```python
from build123d import *

# Parameters (mm, degrees)
MAIN_FEATURES_SKETCH_W   = 70.04
MAIN_FEATURES_SKETCH_H   = 57.05
MAIN_BODY_DEPTH          = 27.3
WIRES_START              = 2.1
MAIN_FEATURES_SKETCH_3_W = 4
MAIN_FEATURES_SKETCH_3_H = 10
WIRES_2_DEPTH            = 4
LENS_CUTOUT_START        = 27.3
MAIN_FEATURES_SKETCH_4_W = 50
MAIN_FEATURES_SKETCH_4_H = 37
LENS_CUTOUT_DEPTH        = 3.1
MAIN_FEATURES_SKETCH_5_R = 2.25
SCREW_HEADS_DEPTH        = 0.3
FILLET1_R                = 1
FILLET2_R                = 2


with BuildPart() as part:
    # main_features_sketch → main_body (new body)
    with BuildSketch(Plane.XY):
        Rectangle(MAIN_FEATURES_SKETCH_W, MAIN_FEATURES_SKETCH_H)
    extrude(amount=MAIN_BODY_DEPTH)

    # main_features_sketch<3> → wires 2 (add)
    with BuildSketch(Plane.XY.offset(WIRES_START)):
        with Locations((-18, -33.525)):
            Rectangle(MAIN_FEATURES_SKETCH_3_W, MAIN_FEATURES_SKETCH_3_H)
        with Locations((18, -33.525)):
            Rectangle(MAIN_FEATURES_SKETCH_3_W, MAIN_FEATURES_SKETCH_3_H)
    extrude(amount=WIRES_2_DEPTH)

    # main_features_sketch<4> → lens_cutout (cut)
    with BuildSketch(Plane.XY.offset(LENS_CUTOUT_START)):
        Rectangle(MAIN_FEATURES_SKETCH_4_W, MAIN_FEATURES_SKETCH_4_H)
    extrude(amount=-LENS_CUTOUT_DEPTH, mode=Mode.SUBTRACT)

    # main_features_sketch<5> → screw_heads (add)
    with BuildSketch(Plane.XY):
        with Locations((-32, -25.5)):
            Circle(MAIN_FEATURES_SKETCH_5_R)
        with Locations((32, -25.5)):
            Circle(MAIN_FEATURES_SKETCH_5_R)
        with Locations((32, 25.5)):
            Circle(MAIN_FEATURES_SKETCH_5_R)
        with Locations((-32, 25.5)):
            Circle(MAIN_FEATURES_SKETCH_5_R)
    extrude(amount=-SCREW_HEADS_DEPTH)

    # Fillet1
    fillet1_edges = [part.edges().sort_by_distance(p)[0] for p in [
        (35.02, 28.525, 13.65),
        (35.02, -28.525, 13.65),
        (-35.02, -28.525, 13.65),
        (-35.02, 28.525, 13.65),
    ]]
    fillet(fillet1_edges, radius=FILLET1_R)

    # Fillet2
    fillet2_edges = [part.edges().sort_by_distance(p)[0] for p in [
        (20, -33.525, 2.1),
        (20, -33.525, 6.1),
        (16, -33.525, 2.1),
        (16, -33.525, 6.1),
        (-16, -33.525, 2.1),
        (-16, -33.525, 6.1),
        (-20, -33.525, 2.1),
        (-20, -33.525, 6.1),
    ]]
    fillet(fillet2_edges, radius=FILLET2_R - 0.0001)  # a hair under: the kernel refuses the full size


solid = part.part
```
For this review, take the finished solid that the model builds, in its own axes (mm). A direction names the side the tool comes from. Coordinates: 2 decimals unless noted, no trailing zeros. Order: outer loops, then holes, each group sorted by start corner. A loop starts at its lowest first (then second) coordinate and runs counter-clockwise, first axis right, second up. Notation, with made-up numbers: (25.25, -4) - (62.25, -4) arc R21 ccw to (62.25, 24) - close; hole circle Ø4 at (61, -13). An arc over 180 degrees is marked (long way). Answer as a JSON object with one key per item and string values. Group by question number.
1. We need section B-B on x = 1. State the section outline as (y, z) points (3 decimals).
2. We need section C-C on z = 10. State the section outline as (x, y) points (3 decimals).
3. We need section D-D on x = -32. State the section outline as (y, z) points (3 decimals).
4. For probe 1 along Y at (x, z) = (-15, 24.25) (3 decimals); probe 2 along Z at (x, y) = (-22, 7.5); probe 3 along Y at (x, z) = (17.5, 16) (3 decimals), list the stretches that pass through material, from the lowest coordinate up.
5. For faces 1 (the flat face through (0, 0, 0)), 2 (the flat face through (0, 0, 24.2)), 3 (the cylindrical face through (19.43, -33.46, 2.7)), 4 (the cylindrical face through (-16.57, -33.46, 2.7)), list the 3-axis set-ups (+Z, -Z, +X, -X, +Y, -Y) from which the entire face can be reached by the end or side of a thin tool; tool diameter is ignored.
6. Clearance check with flat-ended pins moving along their axes: P1, Ø10, axis at x = 12, z = 14, coming from the -Y side (3 decimals); P2, Ø18.5, axis at x = 8.5, y = -5.5, coming from the +Z side. State where each tip first meets the part, or that it passes through.
7. The part is to be moulded in two halves that separate along Y. For faces 5 (the cylindrical face through (16.57, -33.46, 5.5)), 6 (the flat face through (18, -38.525, 4)), 7 (the flat face through (25, 0, 26)), say which applies: pulls with the +Y half, pulls with the -Y half, needs draft (parallel to the pull), parting line crosses it, or undercut.
Final values:
{
 "1": {"outline": "(-28.525, 0) - (28.525, 0) - (28.525, 27.3) - (18.5, 27.3) - (18.5, 24.2) - (-18.5, 24.2) - (-18.5, 27.3) - (-28.525, 27.3) - close"},
 "2": {"outline": "(-35.02, -27.525) arc R1 ccw to (-34.02, -28.525) - (34.02, -28.525) arc R1 ccw to (35.02, -27.525) - (35.02, 27.525) arc R1 ccw to (34.02, 28.525) - (-34.02, 28.525) arc R1 ccw to (-35.02, 27.525) - close"},
 "3": {"outline": "(-28.525, 0) - (-27.75, 0) - (-27.75, -0.3) - (-23.25, -0.3) - (-23.25, 0) - (23.25, 0) - (23.25, -0.3) - (27.75, -0.3) - (27.75, 0) - (28.525, 0) - (28.525, 27.3) - (-28.525, 27.3) - close"},
 "4": {"probe 1": "-28.525 to -18.5, 18.5 to 28.525", "probe 2": "0 to 24.2", "probe 3": "-28.525 to 28.525"},
 "5": {"face 1": "-Z", "face 2": "+Z", "face 3": "-Z, +X, -Y", "face 4": "-Z, -Y"},
 "6": {"P1": "y = -28.525", "P2": "z = 24.2"},
 "7": {"face 5": "needs draft", "face 6": "pulls with the -Y half", "face 7": "undercut"}
}
